Check sheet for the modelled part. Datum: model origin and axes. Units: mm. Round coordinates to 2 decimals unless told otherwise and drop trailing zeros. Write each loop counter-clockwise with the first axis right and the second up, starting at its lowest first coordinate (ties: lowest second). Pieces come first, ordered by that corner, then holes. Notation, with made-up numbers: (13.5, -15) -> (28.5, -15) arc R26 ccw to (28.5, 23) -> close; hole circle Ø10 at (-6, -17). An arc over 180 degrees is marked (long way). Write item = value, one per line.
from build123d import *

# Parameters (mm, degrees)
SKETCH2_W           = 150
SKETCH2_H           = 20
BOSS_EXTRUDE1_DEPTH = 3
SKETCH3_R           = 5
CUT_EXTRUDE1_DEPTH  = 152.35719342
SKETCH4_R           = 5
CUT_EXTRUDE2_DEPTH  = 152.35719342
FILLET1_R           = 10
FILLET2_R           = 10


with BuildPart() as part:
    # Sketch2 → Boss-Extrude1 (new body)
    with BuildSketch(Plane(origin=(0, 0, 0), x_dir=(1, 0, 0), z_dir=(0, 1, 0))):
        with Locations((75, 10)):
            Rectangle(SKETCH2_W, SKETCH2_H)
    extrude(amount=BOSS_EXTRUDE1_DEPTH)

    # Sketch3 → Cut-Extrude1 (cut, through all)
    with BuildSketch(Plane(origin=(0, 3, 0), x_dir=(1, 0, 0), z_dir=(0, 1, 0))):
        with Locations(Location((9, 10, 0), (0, 0, 270))):
            Circle(SKETCH3_R)
    extrude(amount=-CUT_EXTRUDE1_DEPTH, mode=Mode.SUBTRACT)

    # Sketch4 → Cut-Extrude2 (cut, through all)
    with BuildSketch(Plane(origin=(0, 3, 0), x_dir=(1, 0, 0), z_dir=(0, 1, 0))):
        with Locations(Location((141, 10, 0), (0, 0, 270))):
            Circle(SKETCH4_R)
    extrude(amount=-CUT_EXTRUDE2_DEPTH, mode=Mode.SUBTRACT)

    # Fillet1
    fillet1_edges = [part.edges().sort_by_distance(p)[0] for p in [
        (0, 1.5, -20),
        (0, 1.5, 0),
    ]]
    fillet(fillet1_edges, radius=FILLET1_R - 0.0001)  # a hair under: the kernel refuses the full size

    # Fillet2
    fillet2_edges = [part.edges().sort_by_distance(p)[0] for p in [
        (150, 1.5, -20),
        (150, 1.5, 0),
    ]]
    fillet(fillet2_edges, radius=FILLET2_R - 0.0001)  # a hair under: the kernel refuses the full size


solid = part.part
(1) Material ranges on L1, parallel to X at y = 1.7, z = -10; L2, parallel to X at y = 2.7, z = -10.75; L3, parallel to Z at x = 12, y = 1.8, recorded low to high. Write a range as [from, to].
Worked answers:
L1 = [0, 4], [14, 136], [146, 150]
L2 = [0.03, 4.06], [13.94, 136.06], [145.94, 149.97]
L3 = [-20, -14], [-6, 0]
(2) Release check for a two-part mould opening along X. For faces 1 (the cylindrical face through (146.99, 1.52, -17.15)), 2 (the cylindrical face through (10.5, 1.52, -5.23)), 3 (the flat face through (74, 1, -20)), 4 (the cylindrical face through (136.564, 1.521, -7.693)) record: pulls with the +X half, pulls with the -X half, needs draft (parallel to the pull), parting line crosses it, or undercut.
Worked answers:
face_1 = pulls with the +X half
face_2 = undercut
face_3 = needs draft
face_4 = undercut
(3) Sectioned sample at B-B on y = 0.7. Count the separate pieces of the cut face and the enclosed holes in it, then the cut area to 3 significant figures.
Worked answers:
separate_pieces = 1
enclosed_holes = 2
area = 2,760 mm²
(4) Go/stop test with a flat-tipped pin: P1, Ø11.5, axis at x = 141, z = -10, coming from the -Y side. Record where the tip stops, or that it passes through.
Worked answers:
P1 = 0
(5) Sectioned sample at A-A on z = -6.75. Enter the section's corners in (x, y), then the cut area to 3 significant figures.
Worked answers:
outline = (0.54, 0) -> (5.2, 0) -> (5.2, 3) -> (0.54, 3) -> close; (12.8, 0) -> (137.2, 0) -> (137.2, 3) -> (12.8, 3) -> close; (144.8, 0) -> (149.46, 0) -> (149.46, 3) -> (144.8, 3) -> close
area = 401 mm²
